Can you work these out from the model? Positions are in its coordinate system, mm. Give positions to 0.01 mm unless a question says otherwise; leave off trailing zeros. Write each loop counter-clockwise with the first axis right and the second up, starting at its lowest first coordinate (ties: lowest second). Pieces come first, ordered by that corner, then holes. Notation, with made-up numbers: (54.25, 46.5) - (63.25, 46.5) arc R24 ccw to (63.25, 65.5) - close; hole circle Ø3 at (87, 41.5). An arc over 180 degrees is marked (long way). Use a Markdown table: item, result. Add a question column.
```python
from build123d import *

# Parameters (mm, degrees)
SKETCH1_R           = 1.55
SKETCH1_W           = 52
SKETCH1_H           = 15
SKETCH1_W_2         = 50
SKETCH1_H_2         = 45
BOSS_EXTRUDE1_DEPTH = 5


with BuildPart() as part:
    # Sketch1 → Boss-Extrude1 (new body)
    with BuildSketch(Plane(origin=(0, 0, 0), x_dir=(1, 0, 0), z_dir=(0, 1, 0))):
        Polygon((90, 30), (97, 30), (97, -30), (90, -30), (90, -82.5), (-90, -82.5), (-90, -30), (-97, -30), (-97, 30), (-90, 30), (-90, 89.5), (90, 89.5), align=None)
        with Locations((70, 19.5)):
            Circle(SKETCH1_R, mode=Mode.SUBTRACT)
        with Locations((-70, 19.5)):
            Circle(SKETCH1_R, mode=Mode.SUBTRACT)
        with Locations((0, 72)):
            Rectangle(SKETCH1_W, SKETCH1_H, mode=Mode.SUBTRACT)
        with Locations((-40, -42)):
            Rectangle(SKETCH1_W_2, SKETCH1_H_2, mode=Mode.SUBTRACT)
        with Locations((40, -42)):
            Rectangle(SKETCH1_W_2, SKETCH1_H_2, mode=Mode.SUBTRACT)
    extrude(amount=BOSS_EXTRUDE1_DEPTH)


solid = part.part
```
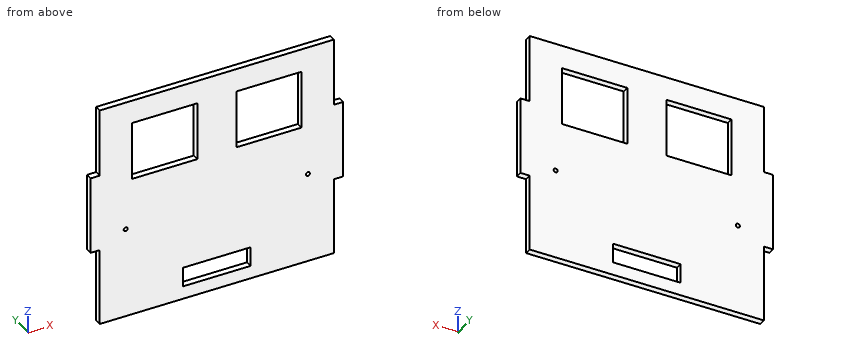
Q1. I'm going to push flat-ended pins straight in: P1, Ø1.5, axis at y = 2, z = -72, coming from the +X side; P2, Ø2.5, axis at x = -70, z = -19.5, coming from the +Y side; P3, Ø1.5, axis at x = 94, y = 1.5, coming from the -Z side; P4, Ø2, axis at y = 2.5, z = -65, coming from the -X side. Where does each tip first touch, or does it pass through?
Q2. Suppose I cut it at B-B (z = 62). Please give me the cut outline in (x, y).
Q3. Suppose I cut it at C-C (y = 2.15). Please give me the cut outline in (x, z).
Q4. If I drill on probe 1 along Z at (x, y) = (25, 0.4); probe 2 along X at (y, z) = (3.35, 22); probe 3 along X at (y, z) = (2.9, -19.5), over which ranges is the centre line in solid material (lowest first)? Write a range as [from, to].
Q5. Suppose I cut it at A-A (x = -48.5). Please give me the cut outline in (y, z), and give its area (3 significant figures).
Derived:
| question | item | result |
|---|---|---|
| 1 | P1 | x = 90 |
| 1 | P2 | through |
| 1 | P3 | z = -30 |
| 1 | P4 | x = -90 |
| 2 | outline | (-90, 0) - (-65, 0) - (-65, 5) - (-90, 5) - close; (-15, 0) - (15, 0) - (15, 5) - (-15, 5) - close; (65, 0) - (90, 0) - (90, 5) - (65, 5) - close |
| 3 | outline | (-97, -30) - (-90, -30) - (-90, -89.5) - (90, -89.5) - (90, -30) - (97, -30) - (97, 30) - (90, 30) - (90, 82.5) - (-90, 82.5) - (-90, 30) - (-97, 30) - close; hole circle Ø3.1 at (-70, -19.5); hole (-65, 19.5) - (-15, 19.5) - (-15, 64.5) - (-65, 64.5) - close; hole (-26, -79.5) - (26, -79.5) - (26, -64.5) - (-26, -64.5) - close; hole (15, 19.5) - (65, 19.5) - (65, 64.5) - (15, 64.5) - close; hole circle Ø3.1 at (70, -19.5) |
| 4 | probe 1 | [-89.5, -79.5], [-64.5, 19.5], [64.5, 82.5] |
| 4 | probe 2 | [-97, -65], [-15, 15], [65, 97] |
| 4 | probe 3 | [-97, -71.55], [-68.45, 68.45], [71.55, 97] |
| 5 | outline | (0, -89.5) - (5, -89.5) - (5, 19.5) - (0, 19.5) - close; (0, 64.5) - (5, 64.5) - (5, 82.5) - (0, 82.5) - close |
| 5 | area | 635 mm² |
